```python
from build123d import *

# Parameters (mm, degrees)
SKETCH1_W               = 84
SKETCH1_H               = 78
BOSS_EXTRUDE1_DEPTH     = 4.5
FILLET2_R               = 2
CUT_EXTRUDE1_DEPTH      = 69.558369292
CUT_EXTRUDE1_DEPTH_BACK = 69.558369292
BOSS_EXTRUDE2_DEPTH     = 48.5
FILLET4_R               = 2
RIB7_REACH              = 115.053
SKETCH4_WALL_W          = 281.181587792
SKETCH4_WALL_H          = 3
RIB8_REACH              = 93.81
SKETCH6_WALL_W          = 238.694589152
SKETCH6_WALL_H          = 3
SKETCH7_R               = 11.5
SKETCH7_R_2             = 1.5
CUT_EXTRUDE2_DEPTH      = 101.244700608
SKETCH8_W               = 15
SKETCH8_H               = 14
BOSS_EXTRUDE3_DEPTH     = 20
FILLET5_R               = 7
FILLET6_R               = 2
SKETCH9_R               = 4
CUT_EXTRUDE3_DEPTH      = 10
CUT_EXTRUDE4_DEPTH      = 84.858511792


with BuildPart() as part:
    # Sketch1 → Boss-Extrude1 (new body)
    with BuildSketch(Plane(origin=(0, 0, 0), x_dir=(1, 0, 0), z_dir=(0, 1, 0))):
        with Locations((0, -15)):
            Rectangle(SKETCH1_W, SKETCH1_H)
    extrude(amount=BOSS_EXTRUDE1_DEPTH)

    # Fillet2
    fillet2_edges = [part.edges().sort_by_distance(p)[0] for p in [
        (-42, 2.25, -24),
        (42, 2.25, -24),
        (42, 2.25, 54),
        (-42, 2.25, 54),
    ]]
    fillet(fillet2_edges, radius=FILLET2_R)

    # Sketch2 → Cut-Extrude1 (cut, two sides)
    with BuildSketch(Plane(origin=(0, 4.5, 0), x_dir=(1, 0, 0), z_dir=(0, 1, 0))) as cut_extrude1_sk:
        with BuildLine():
            Line((-33.5, -16.749999598), (-33.5, -45.249999598))
            ThreePointArc((-33.5, -45.249999598), (-30.750000201, -48), (-28, -45.25))
            Line((-28, -45.25), (-28, -16.749999598))
            ThreePointArc((-28, -16.749999598), (-30.75, -13.999999598), (-33.5, -16.749999598))
        make_face()
        with BuildLine():
            Line((2.5, -16.749999598), (2.5, -45.249999598))
            ThreePointArc((2.5, -45.249999598), (-0.249999799, -48), (-3, -45.25))
            Line((-3, -45.25), (-3, -16.749999598))
            ThreePointArc((-3, -16.749999598), (-0.25, -13.999999598), (2.5, -16.749999598))
        make_face()
    extrude(amount=CUT_EXTRUDE1_DEPTH, mode=Mode.SUBTRACT)
    extrude(cut_extrude1_sk.sketch, amount=-CUT_EXTRUDE1_DEPTH_BACK, mode=Mode.SUBTRACT)

    # Sketch3 → Boss-Extrude2 (add)
    with BuildSketch(Plane(origin=(0, 4.5, 0), x_dir=(1, 0, 0), z_dir=(0, 1, 0))):
        with BuildLine():
            Line((-42, 20), (10, 20))
            Line((10, 20), (10, 24))
            Line((10, 24), (-40, 24))
            ThreePointArc((-40, 24), (-41.414213562, 23.414213562), (-42, 22))
            Line((-42, 22), (-42, 20))
        make_face()
    extrude(amount=BOSS_EXTRUDE2_DEPTH)

    # Fillet4
    fillet4_edges = [part.edges().sort_by_distance(p)[0] for p in [
        (-42, 53, -21),
        (10, 53, -22),
        (-15, 53, -24),
        (-41.414213562, 53, -23.414213562),
    ]]
    fillet(fillet4_edges, radius=FILLET4_R)

    # Sketch4 wall → Rib7 (add, up to next)
    with BuildSketch(Plane(origin=(-42, 24, -2), x_dir=(0, 0.734803444627, -0.678280102733), z_dir=(0, -0.678280102733, -0.734803444627)), mode=Mode.PRIVATE) as rib7_sk1:
        with Locations((0, 1.5)):
            Rectangle(SKETCH4_WALL_W, SKETCH4_WALL_H)
    rib7_tool1 = extrude(rib7_sk1.sketch, amount=RIB7_REACH, mode=Mode.PRIVATE) - part.part
    add(rib7_tool1.solids().sort_by_distance((-42, 24, -2))[0])

    # Sketch6 wall → Rib8 (add, up to next)
    with BuildSketch(Plane(origin=(10, 24, -2), x_dir=(0, -0.734803444627, 0.678280102733), z_dir=(0, -0.678280102733, -0.734803444627)), mode=Mode.PRIVATE) as rib8_sk1:
        with Locations((0, 1.5)):
            Rectangle(SKETCH6_WALL_W, SKETCH6_WALL_H)
    rib8_tool1 = extrude(rib8_sk1.sketch, amount=RIB8_REACH, mode=Mode.PRIVATE) - part.part
    add(rib8_tool1.solids().sort_by_distance((10, 24, -2))[0])

    # Sketch7 → Cut-Extrude2 (cut, through all)
    with BuildSketch(Plane.XY.offset(-20)):
        with Locations((-16.25, 25.65)):
            Circle(SKETCH7_R)
        with Locations((-31.75, 41.5)):
            Circle(SKETCH7_R_2)
        with Locations((-31.75, 10.5)):
            Circle(SKETCH7_R_2)
        with Locations(Location((-0.75, 10.5, 0), (0, 0, 180))):
            Circle(SKETCH7_R_2)
        with Locations(Location((-0.75, 41.5, 0), (0, 0, 180))):
            Circle(SKETCH7_R_2)
    extrude(amount=-CUT_EXTRUDE2_DEPTH, mode=Mode.SUBTRACT)

    # Sketch8 → Boss-Extrude3 (add)
    with BuildSketch(Plane(origin=(0, 4.5, 0), x_dir=(1, 0, 0), z_dir=(0, 1, 0))):
        with Locations((27, 10)):
            Rectangle(SKETCH8_W, SKETCH8_H)
    extrude(amount=BOSS_EXTRUDE3_DEPTH)

    # Fillet5
    fillet5_edges = [part.edges().sort_by_distance(p)[0] for p in [
        (19.5, 4.5, -10),
        (34.5, 4.5, -10),
    ]]
    fillet(fillet5_edges, radius=FILLET5_R)

    # Fillet6
    fillet6_edges = [part.edges().sort_by_distance(p)[0] for p in [
        (19.5, 24.5, -10),
        (34.5, 24.5, -10),
    ]]
    fillet(fillet6_edges, radius=FILLET6_R)

    # Sketch9 → Cut-Extrude3 (cut)
    with BuildSketch(Plane(origin=(0, 0, -17), x_dir=(-1, 0, 0), z_dir=(0, 0, -1))):
        with Locations((-27, 16.5)):
            Circle(SKETCH9_R)
    extrude(amount=-CUT_EXTRUDE3_DEPTH, mode=Mode.SUBTRACT)

    # Sketch10 → Cut-Extrude4 (cut, through all)
    with BuildSketch(Plane(origin=(0, 4.5, 0), x_dir=(1, 0, 0), z_dir=(0, 1, 0))):
        with BuildLine():
            Line((24.25, -32.75), (24.25, -45.25))
            ThreePointArc((24.25, -45.25), (26.999999703, -48), (29.75, -45.250000593))
            Line((29.75, -45.250000593), (29.75, -32.749975496))
            ThreePointArc((29.75, -32.749975496), (26.999987748, -29.999987748), (24.25, -32.75))
        make_face()
    extrude(amount=-CUT_EXTRUDE4_DEPTH, mode=Mode.SUBTRACT)


solid = part.part
```
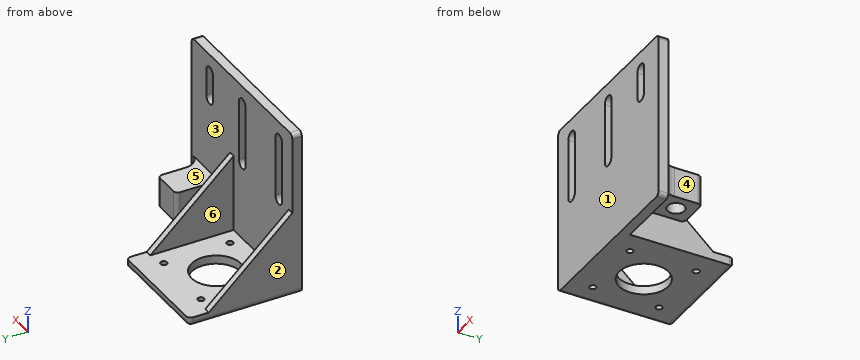
CAD build for the part. Positions are in the model's coordinates, mm. Face numbers are marked on the shaded views. A direction names the side the tool comes from. Give positions to 0.01 mm unless a question says otherwise; leave off trailing zeros. Order: outer loops, then holes, each group sorted by start corner. A loop starts at its lowest first (then second) coordinate and runs counter-clockwise, first axis right, second up.
(1) Saw through at D-D, the plane x = -36. Give the cut face in (y, z), then the cut area to 3 significant figures.
(2) Saw through at C-C, the plane y = 41.5. Give the cut face in (x, z), then the cut area to 3 significant figures.
(3) Mould opens along X. For the marked faces 1, 2 and 3 say: released by +X, released by -X, zero draft, split by the parting line, or undercut.
(4) Flat gauge pins, fed straight in: pin 1 (1.5 mm diameter, centred on x = 5.5, y = 15.5, fed in from +Z); pin 2 (5.5 mm diameter, centred on x = 29.5, z = -9.5, fed in from +Y); pin 3 (10.5 mm diameter, centred on x = 27, y = 16.5, fed in from -Z). Where does each tip first touch, or does it go through?
(5) Saw through at B-B, the plane x = -16.25. Give the cut face in (y, z), then the cut area to 3 significant figures.
(6) Drill centre lines: L1, parallel to X at y = 8, z = -6; L2, parallel to Y at x = -16, z = -21; L3, parallel to X at y = 10, z = -21. Where is each one in solid material? Low to high.
(7) Tool access for the marked faces 4, 5 and 6: list every direction of +Z, -Z, +X, -X, +Y, -Y with a clear straight run to the whole face (end or side of a thin tool).
(8) Saw through at A-A, the plane z = 41.5. Give the cut face in (x, y).
Results found:
1. outline: (0, -24) - (51, -24) arc R2 ccw to (53, -22) - (53, -20) - (4.5, -20) - (4.5, 54) - (0, 54) - close
1. area: 544 mm2
2. outline: (-42, -22) arc R2 ccw to (-40, -24) - (-33.25, -24) - (-33.25, -20) - (-39, -20) - (-39, -18.15) - (-42, -18.15) - close; (-30.25, -24) - (-2.25, -24) - (-2.25, -20) - (-30.25, -20) - close; (0.75, -24) - (10, -24) - (10, -18.15) - (7, -18.15) - (7, -20) - (0.75, -20) - close
2. area: 194 mm2
3. face 1: zero draft
3. face 2: released by -X
3. face 3: undercut
4. pin 1: stops at z = -20
4. pin 2: stops at y = 24.5
4. pin 3: stops at z = -17
5. outline: (0, -24) - (14.15, -24) - (14.15, -20) - (4.5, -20) - (4.5, 54) - (0, 54) - close; (37.15, -24) - (51, -24) arc R2 ccw to (53, -22) - (53, -20) - (37.15, -20) - close
5. area: 452 mm2
6. L1: x = -42 to -39, 7 to 10, 18.56 to 35.44
6. L2: y = 0 to 14.15, 37.15 to 53
6. L3: x = -42 to -33.16, -30.34 to -2.16, 0.66 to 10
7. face 4: +Z, -Z, +X, +Y
7. face 5: +Z, +X, +Y
7. face 6: +Z, +Y
8. outline: (-42, 0) - (-33.5, 0) - (-33.5, 4.5) - (-42, 4.5) - close; (-28, 0) - (-3, 0) - (-3, 4.5) - (-28, 4.5) - close; (2.5, 0) - (24.25, 0) - (24.25, 4.5) - (2.5, 4.5) - close; (29.75, 0) - (42, 0) - (42, 4.5) - (29.75, 4.5) - close
